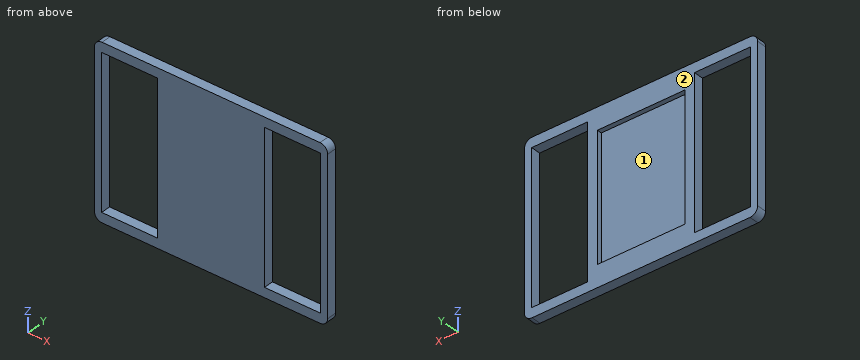
```python
from build123d import *

# Parameters (mm, degrees)
SKETCH1_W           = 304.8
SKETCH1_H           = 222.25
BOSS_EXTRUDE1_DEPTH = 12.7
SKETCH2_W           = 73.025
SKETCH2_H           = 196.85
CUT_EXTRUDE1_DEPTH  = 12.7
SKETCH3_W           = 114.3
SKETCH3_H           = 165.1
CUT_EXTRUDE2_DEPTH  = 6.35
FILLET1_R           = 10


with BuildPart() as part:
    # Sketch1 → Boss-Extrude1 (new body)
    with BuildSketch(Plane(origin=(0, 0, 0), x_dir=(1, 0, 0), z_dir=(0, 1, 0))):
        with Locations((157.198920378, 111.125)):
            Rectangle(SKETCH1_W, SKETCH1_H)
    extrude(amount=BOSS_EXTRUDE1_DEPTH)

    # Sketch2 → Cut-Extrude1 (cut)
    with BuildSketch(Plane(origin=(0, 12.7, 0), x_dir=(1, 0, 0), z_dir=(0, 1, 0))):
        with Locations((50.836420378, 111.125)):
            Rectangle(SKETCH2_W, SKETCH2_H)
        with Locations((263.561420378, 111.125)):
            Rectangle(SKETCH2_W, SKETCH2_H)
    extrude(amount=-CUT_EXTRUDE1_DEPTH, mode=Mode.SUBTRACT)

    # Sketch3 → Cut-Extrude2 (cut)
    with BuildSketch(Plane(origin=(0, 12.7, 0), x_dir=(1, 0, 0), z_dir=(0, 1, 0))):
        with Locations((157.123394244, 111.125)):
            Rectangle(SKETCH3_W, SKETCH3_H)
    extrude(amount=-CUT_EXTRUDE2_DEPTH, mode=Mode.SUBTRACT)

    # Fillet1
    fillet1_edges = [part.edges().sort_by_distance(p)[0] for p in [
        (4.798920378, 6.35, -222.25),
        (309.598920378, 6.35, -222.25),
        (309.598920378, 6.35, 0),
        (4.798920378, 6.35, 0),
    ]]
    fillet(fillet1_edges, radius=FILLET1_R)


solid = part.part
```
The model under review builds one solid part; all positions refer to its coordinate system, in mm. Face numbers are marked on the shaded views. A direction names the side the tool comes from. Round coordinates to 2 decimals unless told otherwise and drop trailing zeros. Order: outer loops, then holes, each group sorted by start corner. A loop starts at its lowest first (then second) coordinate and runs counter-clockwise, first axis right, second up. Notation, with made-up numbers: M 20,43 L 32,43 A29 ccw 32,78 Z; hole C 23,-9.75 d10. An arc over 180 degrees is marked long. Use a Markdown table: item, result.
1) Consider section D-D (x = 193). Write out the cut boundary in (y, z) (3 decimals).
Report:
| item | result |
|---|---|
| outline | M 0,-222.25 L 12.7,-222.25 L 12.7,-193.675 L 6.35,-193.675 L 6.35,-28.575 L 12.7,-28.575 L 12.7,0 L 0,0 Z |
2) Insertion check: pin 1 (1 mm diameter, centred on x = 218.5, z = -118.5, fed in from -Y). The pin has a flat end and moves straight along its axis. Give the tip position at first contact, or say it passes through.
Report:
| item | result |
|---|---|
| pin 1 | y = 0 |
3) Consider section A-A (z = -125.5). Write out the cut boundary in (x, y).
Report:
| item | result |
|---|---|
| outline | M 4.8,0 L 14.32,0 L 14.32,12.7 L 4.8,12.7 Z; M 87.35,0 L 227.05,0 L 227.05,12.7 L 214.27,12.7 L 214.27,6.35 L 99.97,6.35 L 99.97,12.7 L 87.35,12.7 Z; M 300.07,0 L 309.6,0 L 309.6,12.7 L 300.07,12.7 Z |
4) Tool access review of the marked faces 1 and 2: name each direction out of +Z, -Z, +X, -X, +Y, -Y from which nothing blocks a thin tool from reaching the whole face with its end or side.
Report:
| item | result |
|---|---|
| face 1 | +Y |
| face 2 | +Z, -Z, +X, -X, +Y |
5) Wall thickness on line 1 along X through (y, z) = (8, -200.5); line 2 along X through (y, z) = (7.75, -158.5); line 3 along Z through (x, y) = (235, 2.75): over which ranges is each line inside the solid? List them lowest first. Write a range as [from, to].
Report:
| item | result |
|---|---|
| line 1 | [4.8, 14.32], [87.35, 227.05], [300.07, 309.6] |
| line 2 | [4.8, 14.32], [87.35, 99.97], [214.27, 227.05], [300.07, 309.6] |
| line 3 | [-222.25, -209.55], [-12.7, 0] |
6) Consider section C-C (y = 3.5). Write out the cut boundary in (x, z).
Report:
| item | result |
|---|---|
| outline | M 4.8,-212.25 A10 ccw 14.8,-222.25 L 299.6,-222.25 A10 ccw 309.6,-212.25 L 309.6,-10 A10 ccw 299.6,0 L 14.8,0 A10 ccw 4.8,-10 Z; hole M 14.32,-209.55 L 87.35,-209.55 L 87.35,-12.7 L 14.32,-12.7 Z; hole M 227.05,-209.55 L 300.07,-209.55 L 300.07,-12.7 L 227.05,-12.7 Z |
7) Consider section B-B (x = 62). Write out the cut boundary in (y, z).
Report:
| item | result |
|---|---|
| outline | M 0,-222.25 L 12.7,-222.25 L 12.7,-209.55 L 0,-209.55 Z; M 0,-12.7 L 12.7,-12.7 L 12.7,0 L 0,0 Z |
